from build123d import *

# Parameters (mm, degrees)
F0_W      = 50
F0_H      = 10
F1_DEPTH  = 60
F2_W      = 50
F2_H      = 10
F3_DEPTH  = 10
F4_W      = 50
F4_H      = 10
F5_DEPTH  = 20
F6_W      = 50
F6_H      = 10
F7_DEPTH  = 30
F8_W      = 50
F8_H      = 10
F9_DEPTH  = 40
F10_W     = 50
F10_H     = 10
F11_DEPTH = 50


with BuildPart() as f1:
    # F0 (on Top) → F1 (new body)
    with BuildSketch(Plane.XY):
        Rectangle(F0_W, F0_H)
    extrude(amount=F1_DEPTH)

    # F2 (on face) → F3 (join)
    with BuildSketch(Plane.XZ.offset(5)):
        with Locations((0, 45)):
            Rectangle(F2_W, F2_H)
    extrude(amount=F3_DEPTH)

    # F4 (on face) → F5 (join)
    with BuildSketch(Plane.XZ.offset(5)):
        with Locations((0, 35)):
            Rectangle(F4_W, F4_H)
    extrude(amount=F5_DEPTH)

    # F6 (on face) → F7 (join)
    with BuildSketch(Plane.XZ.offset(5)):
        with Locations((0, 25)):
            Rectangle(F6_W, F6_H)
    extrude(amount=F7_DEPTH)

    # F8 (on face) → F9 (join)
    with BuildSketch(Plane.XZ.offset(5)):
        with Locations((0, 15)):
            Rectangle(F8_W, F8_H)
    extrude(amount=F9_DEPTH)

    # F10 (on face) → F11 (join)
    with BuildSketch(Plane.XZ.offset(5)):
        with Locations((0, 5)):
            Rectangle(F10_W, F10_H)
    extrude(amount=F11_DEPTH)


solid = f1.part
Geometry check sheet. Reference: the model listing, model coordinates, mm. A direction names the side the tool comes from. Round coordinates to 2 decimals unless told otherwise and drop trailing zeros. Loops run counter-clockwise (first coordinate to the right, second up) from the corner with the lowest first, then second, coordinate; pieces in that order, holes last.
Item 1: Gauge pin test, flat ends, axial feed: pin 1 (2 mm diameter, centred on x = 14.5, y = -44.5, fed in from +Z); pin 2 (2 mm diameter, centred on x = -5.5, z = 17, fed in from -Y); pin 3 (11 mm diameter, centred on x = 1.5, z = 56, fed in from -Y); pin 4 (8 mm diameter, centred on y = -17, z = 54, fed in from -X). Record the tip position at first contact, or that the pin passes through.
Item 2: Access from +Z, -Z, +X, -X, +Y, -Y to the whole of each face (thin tool, end or side, straight path). Record for faces 1 (the flat face through (0, -25, 0)), 2 (the flat face through (0, -40, 20)).
Item 3: Cross-section at A-A on x = 7.5. Record the boundary of the cut face in (y, z).
Item 4: Mould release check, pull along X, two halves, no side actions. Record for faces 3 (the flat face through (0, -15, 45)), 4 (the flat face through (25, -18, 23)), 5 (the flat face through (-25, -18, 23)): pulls with the +X half, pulls with the -X half, needs draft (parallel to the pull), parting line crosses it, or undercut.
Item 5: Cross-section at B-B on z = 46. Record the boundary of the cut face in (x, y), then the cut area to 3 significant figures.
Item 6: Thickness scan on line 1 (Y direction, x = 17.5, z = 42.5); line 2 (Z direction, x = 14, y = -9); line 3 (Y direction, x = -19, z = 21). Record the ranges inside material, lowest first.
Item 7: Cross-section at C-C on y = -33. Record the boundary of the cut face in (x, z).
Answer sheet:
1. pin 1: stops at z = 20
1. pin 2: stops at y = -45
1. pin 3: stops at y = -5
1. pin 4: passes through
2. face 1: -Z, +X, -X, +Y, -Y
2. face 2: +Z, +X, -X, -Y
3. outline: (-55, 0) - (5, 0) - (5, 60) - (-5, 60) - (-5, 50) - (-15, 50) - (-15, 40) - (-25, 40) - (-25, 30) - (-35, 30) - (-35, 20) - (-45, 20) - (-45, 10) - (-55, 10) - close
4. face 3: needs draft
4. face 4: pulls with the +X half
4. face 5: pulls with the -X half
5. outline: (-25, -15) - (25, -15) - (25, 5) - (-25, 5) - close
5. area: 1,000 mm2
6. line 1: y = -15 to 5
6. line 2: z = 0 to 50
6. line 3: y = -35 to 5
7. outline: (-25, 0) - (25, 0) - (25, 30) - (-25, 30) - close
